```python
from build123d import *

# Parameters (mm, degrees)
SKETCH_2_R          = 2.25
EXTRUDE_2_DEPTH     = 5
SKETCH_3_W          = 25
SKETCH_3_H          = 100
CUT_EXTRUDE_1_DEPTH = 5
CUT_EXTRUDE_2_DEPTH = 5
SKETCH_5_R          = 1.75
SKETCH_5_W          = 15
SKETCH_5_H          = 5
CUT_EXTRUDE_3_DEPTH = 213.190951739
SKETCH_7_R          = 2.25
SKETCH_7_W          = 13
SKETCH_7_H          = 32
SKETCH_7_W_2        = 45
SKETCH_7_H_2        = 70
CUT_EXTRUDE_4_DEPTH = 10
SKETCH_8_R          = 1.75
CUT_EXTRUDE_5_DEPTH = 213.190951739


with BuildPart() as part:
    # 草圖2 → 填料-伸長2 (new body)
    with BuildSketch(Plane(origin=(0, 0, 0), x_dir=(1, 0, 0), z_dir=(0, 1, 0))):
        Polygon((-150, 150), (150, 150), (150, -50), (70, -150), (-70, -150), (-150, -50), align=None)
        with Locations(Location((-105, 121, 0), (0, 0, 270))):
            Circle(SKETCH_2_R, mode=Mode.SUBTRACT)
        with Locations(Location((-105, 79, 0), (0, 0, 270))):
            Circle(SKETCH_2_R, mode=Mode.SUBTRACT)
        with Locations(Location((-55, 79, 0), (0, 0, 270))):
            Circle(SKETCH_2_R, mode=Mode.SUBTRACT)
        with Locations(Location((-55, 121, 0), (0, 0, 270))):
            Circle(SKETCH_2_R, mode=Mode.SUBTRACT)
        with Locations(Location((55, 121, 0), (0, 0, 270))):
            Circle(SKETCH_2_R, mode=Mode.SUBTRACT)
        with Locations(Location((55, 79, 0), (0, 0, 270))):
            Circle(SKETCH_2_R, mode=Mode.SUBTRACT)
        with Locations(Location((105, 121, 0), (0, 0, 270))):
            Circle(SKETCH_2_R, mode=Mode.SUBTRACT)
        with Locations(Location((105, 79, 0), (0, 0, 270))):
            Circle(SKETCH_2_R, mode=Mode.SUBTRACT)
    extrude(amount=EXTRUDE_2_DEPTH)

    # 草圖3 → 除料-伸長1 (cut)
    with BuildSketch(Plane(origin=(0, 5, 0), x_dir=(1, 0, 0), z_dir=(0, 1, 0))):
        with Locations((-137.5, 100)):
            Rectangle(SKETCH_3_W, SKETCH_3_H)
        with Locations((137.5, 100)):
            Rectangle(SKETCH_3_W, SKETCH_3_H)
    extrude(amount=-CUT_EXTRUDE_1_DEPTH, mode=Mode.SUBTRACT)

    # 草圖4 → 除料-伸長2 (cut)
    with BuildSketch(Plane(origin=(0, 5, 0), x_dir=(1, 0, 0), z_dir=(0, 1, 0))):
        with BuildLine():
            Line((-105.5, 45), (-105.5, -15))
            ThreePointArc((-105.5, -15), (-107.5, -17), (-109.5, -15))
            Line((-109.5, -15), (-109.5, 45))
            ThreePointArc((-109.5, 45), (-107.5, 47), (-105.5, 45))
        make_face()
        with BuildLine():
            Line((-74.5, 45), (-74.5, -15))
            ThreePointArc((-74.5, -15), (-72.5, -17), (-70.5, -15))
            Line((-70.5, -15), (-70.5, 45))
            ThreePointArc((-70.5, 45), (-72.5, 47), (-74.5, 45))
        make_face()
        with BuildLine():
            Line((105.5, 45), (105.5, -15))
            ThreePointArc((105.5, -15), (107.5, -17), (109.5, -15))
            Line((109.5, -15), (109.5, 45))
            ThreePointArc((109.5, 45), (107.5, 47), (105.5, 45))
        make_face()
        with BuildLine():
            Line((74.5, 45), (74.5, -15))
            ThreePointArc((74.5, -15), (72.5, -17), (70.5, -15))
            Line((70.5, -15), (70.5, 45))
            ThreePointArc((70.5, 45), (72.5, 47), (74.5, 45))
        make_face()
    extrude(amount=-CUT_EXTRUDE_2_DEPTH, mode=Mode.SUBTRACT)

    # 草圖5 → 除料-伸長3 (cut, through all)
    with BuildSketch(Plane(origin=(0, 5, 0), x_dir=(1, 0, 0), z_dir=(0, 1, 0))):
        with Locations(Location((0, 62, 0), (0, 0, 270))):
            Circle(SKETCH_5_R)
        with Locations(Location((-80, 62, 0), (0, 0, 270))):
            Circle(SKETCH_5_R)
        with Locations(Location((80, 62, 0), (0, 0, 90))):
            Circle(SKETCH_5_R)
        with Locations(Location((80, 138, 0), (0, 0, 270))):
            Circle(SKETCH_5_R)
        with Locations(Location((-80, 138, 0), (0, 0, 90))):
            Circle(SKETCH_5_R)
        with Locations(Location((0, 138, 0), (0, 0, 90))):
            Circle(SKETCH_5_R)
        with Locations((16, 62)):
            Rectangle(SKETCH_5_W, SKETCH_5_H)
        with Locations((-16, 62)):
            Rectangle(SKETCH_5_W, SKETCH_5_H)
        with Locations((-96, 62)):
            Rectangle(SKETCH_5_W, SKETCH_5_H)
        with Locations((-64, 62)):
            Rectangle(SKETCH_5_W, SKETCH_5_H)
        with Locations((64, 62)):
            Rectangle(SKETCH_5_W, SKETCH_5_H)
        with Locations((96, 62)):
            Rectangle(SKETCH_5_W, SKETCH_5_H)
        with Locations((96, 138)):
            Rectangle(SKETCH_5_W, SKETCH_5_H)
        with Locations((64, 138)):
            Rectangle(SKETCH_5_W, SKETCH_5_H)
        with Locations((-64, 138)):
            Rectangle(SKETCH_5_W, SKETCH_5_H)
        with Locations((-96, 138)):
            Rectangle(SKETCH_5_W, SKETCH_5_H)
        with Locations((16, 138)):
            Rectangle(SKETCH_5_W, SKETCH_5_H)
        with Locations((-16, 138)):
            Rectangle(SKETCH_5_W, SKETCH_5_H)
    extrude(amount=-CUT_EXTRUDE_3_DEPTH, mode=Mode.SUBTRACT)

    # 草圖7 → 除料-伸長4 (cut)
    with BuildSketch(Plane(origin=(0, 5, 0), x_dir=(1, 0, 0), z_dir=(0, 1, 0))):
        with Locations(Location((-34.5, -49, 0), (0, 0, 270))):
            Circle(SKETCH_7_R)
        with Locations(Location((-34.5, -91, 0), (0, 0, 270))):
            Circle(SKETCH_7_R)
        with Locations(Location((34.5, -91, 0), (0, 0, 270))):
            Circle(SKETCH_7_R)
        with Locations(Location((34.5, -49, 0), (0, 0, 270))):
            Circle(SKETCH_7_R)
        with Locations((34.5, -70)):
            Rectangle(SKETCH_7_W, SKETCH_7_H)
        with Locations((0, -70)):
            Rectangle(SKETCH_7_W_2, SKETCH_7_H_2)
        with Locations((-34.5, -70)):
            Rectangle(SKETCH_7_W, SKETCH_7_H)
    extrude(amount=-CUT_EXTRUDE_4_DEPTH, mode=Mode.SUBTRACT)

    # 草圖8 → 除料-伸長5 (cut, through all)
    with BuildSketch(Plane(origin=(0, 5, 0), x_dir=(1, 0, 0), z_dir=(0, 1, 0))):
        with Locations(Location((-80, 121, 0), (0, 0, 270))):
            Circle(SKETCH_8_R)
        with Locations(Location((80, 121, 0), (0, 0, 90))):
            Circle(SKETCH_8_R)
        with Locations(Location((-135, -50, 0), (0, 0, 270))):
            Circle(SKETCH_8_R)
        with Locations(Location((-66.283544769, -135.895569039, 0), (0, 0, 270))):
            Circle(SKETCH_8_R)
        with Locations(Location((135, -50, 0), (0, 0, 90))):
            Circle(SKETCH_8_R)
        with Locations(Location((66.283544769, -135.895569039, 0), (0, 0, 90))):
            Circle(SKETCH_8_R)
    extrude(amount=-CUT_EXTRUDE_5_DEPTH, mode=Mode.SUBTRACT)


solid = part.part
```
Check sheet for the modelled part. Datum: model origin and axes. Units: mm. Give positions to 0.01 mm unless a question says otherwise; leave off trailing zeros. Order: outer loops, then holes, each group sorted by start corner. A loop starts at its lowest first (then second) coordinate and runs counter-clockwise, first axis right, second up. Notation, with made-up numbers: M 43.5,83.25 L 73.5,83.25 A17 cw 73.5,110.25 Z; hole C -17,14.5 d11. An arc over 180 degrees is marked long. Answer in a Markdown table with one row per item.
1) Thickness scan on L1, parallel to X at y = 4.6, z = -22.5; L2, parallel to X at y = 3.15, z = -79; L3, parallel to X at y = 3.2, z = 50. Record the ranges inside material, lowest first. Write a range as [from, to].
Filled sheet:
| item | result |
|---|---|
| L1 | x = [-150, -109.5], [-105.5, -74.5], [-70.5, 70.5], [74.5, 105.5], [109.5, 150] |
| L2 | x = [-125, -107.25], [-102.75, -57.25], [-52.75, 52.75], [57.25, 102.75], [107.25, 125] |
| L3 | x = [-150, -136.75], [-133.25, -36.52], [-32.48, -22.5], [22.5, 32.48], [36.52, 133.25], [136.75, 150] |
2) Cross-section at C-C, the plane z = -99. Enter the section's corners in (x, y), plus the area to 3 significant figures.
Filled sheet:
| item | result |
|---|---|
| outline | M -125,0 L 125,0 L 125,5 L -125,5 Z |
| area | 1,250 mm2 |
3) Gauge pin test, flat ends, axial feed: P1, Ø2.5, axis at y = 2.5, z = -106.5, coming from the -X side; P2, Ø1.5, axis at y = 2.5, z = -61, coming from the +X side; P3, Ø2.5, axis at x = 143, y = 2.5, coming from the -Z side; P4, Ø5.5, axis at x = -80, z = -121, coming from the +Y side. Record the tip position at first contact, or that the pin passes through.
Filled sheet:
| item | result |
|---|---|
| P1 | stops at x = -125 |
| P2 | stops at x = 125 |
| P3 | stops at z = -50 |
| P4 | stops at y = 5 |
4) Cross-section at B-B, the plane y = 3.15. Count the separate pieces of the cut face and the enclosed holes in it, plus the area to 3 significant figures.
Filled sheet:
| item | result |
|---|---|
| separate pieces | 1 |
| enclosed holes | 43 |
| area | 70,800 mm2 |
5) Cross-section at A-A, the plane x = 14.5. Enter the section's corners in (y, z).
Filled sheet:
| item | result |
|---|---|
| outline | M 0,-150 L 5,-150 L 5,-140.5 L 0,-140.5 Z; M 0,-135.5 L 5,-135.5 L 5,-64.5 L 0,-64.5 Z; M 0,-59.5 L 5,-59.5 L 5,35 L 0,35 Z; M 0,105 L 5,105 L 5,150 L 0,150 Z |
